Here's how the part is built. I have some questions about the finished solid (model axes, mm). Coordinates: 2 decimals unless noted, no trailing zeros. Write each loop counter-clockwise with the first axis right and the second up, starting at its lowest first coordinate (ties: lowest second). Pieces come first, ordered by that corner, then holes.
Item 1: If we section it at B-B (z = 706.5): Please give me the cut outline in (x, y), then the cut area to 3 significant figures.
Item 2: If I drill on line 1 (Y direction, x = 137, z = 936); line 2 (Y direction, x = 168, z = 928.5), over which ranges is the centre line in solid material (lowest first)?
Item 3: If we section it at A-A (x = 331.5): Please give me the cut outline in (y, z), then the cut area to 3 significant figures.
Item 4: I'm going to push flat-ended pins straight in: pin 1 Ø5 at (x, y) = (225, 2922.5) entering from -Z; pin 2 Ø1.5 at (x, y) = (300.5, 2906.5) entering from -Z; pin 3 Ø3 at (x, z) = (111, 910) entering from +Y. Where does each tip first touch, or does it pass through?
from build123d import *

# Parameters (mm, degrees)
BOSS_EXTRUDE1_DEPTH     = 3
CUT_EXTRUDE2_DEPTH      = 80
BOSS_EXTRUDE2_DEPTH     = 3
SKETCH6_R               = 4.999999998
BOSS_EXTRUDE3_DEPTH     = 3
SKETCH7_R               = 2.099999998
CUT_EXTRUDE8_DEPTH      = 103.727128927
CUT_EXTRUDE8_DEPTH_BACK = 93.470854005


with BuildPart() as part:
    # Sketch1 → Boss-Extrude1 (new body)
    with BuildSketch(Plane(origin=(349.089252495, 2874.058311474, 804.288278977), x_dir=(0.935705749, -0.202672232, 0.288753733), z_dir=(-0.118950757, -0.951829224, -0.282616075))):
        Polygon((-227.79105078, 209.509165447), (-94.070562084, 190.966487567), (-128.879732086, -60.059780262), (-262.600220782, -41.517102382), align=None)
    extrude(amount=-BOSS_EXTRUDE1_DEPTH)

    # Sketch3 → Cut-Extrude2 (cut)
    with BuildSketch(Plane(origin=(688.574610071, 446.833813903, 894.692140277), x_dir=(0.516756682, 0.537673014, -0.66623589), z_dir=(0.567103814, 0.368008283, 0.736860345))):
        Polygon((970.937778761, -219.886702224), (970.937778761, 845.245168422), (-1124.286512281, 775.631358808), (-1124.286512281, -289.500511838), align=None)
    extrude(amount=CUT_EXTRUDE2_DEPTH, mode=Mode.SUBTRACT)

    # Sketch4 → Boss-Extrude2 (add)
    with BuildSketch(Plane(origin=(357.380640452, 2859.715621096, 849.10358184), x_dir=(0.992857215, -0.11667261, -0.024940964), z_dir=(-0.118950757, -0.951829224, -0.282616075))):
        Polygon((-128.234790436, -58.388271423), (-111.076725557, -145.727367265), (1.37386057, -123.636064008), (-4.113952819, -95.701639995), align=None)
    extrude(amount=-BOSS_EXTRUDE2_DEPTH)

    # Sketch6 → Boss-Extrude3 (add)
    with BuildSketch(Plane(origin=(357.737492723, 2862.571108769, 849.951430064), x_dir=(0.992900155, -0.114030405, -0.033857781), z_dir=(0.118950757, 0.951829224, 0.282616075))):
        with Locations((-252.279251986, 111.451515819)):
            Circle(SKETCH6_R)
        with Locations((-137.453856598, 19.622629821)):
            Circle(SKETCH6_R)
        with Locations((-154.05088047, -60.894440309)):
            Circle(SKETCH6_R)
        with Locations((-96.98907211, 70.058139701)):
            Circle(SKETCH6_R)
        with Locations((-34.757829169, 88.136852409)):
            Circle(SKETCH6_R)
        with Locations((-277.861066086, -12.653428287)):
            Circle(SKETCH6_R)
    extrude(amount=-BOSS_EXTRUDE3_DEPTH)

    # Sketch7 → Cut-Extrude8 (cut, two sides)
    with BuildSketch(Plane(origin=(357.737492723, 2862.571108769, 849.951430064), x_dir=(0.992900155, -0.114030405, -0.033857781), z_dir=(0.118950757, 0.951829224, 0.282616075))) as cut_extrude8_sk:
        with Locations((-253.258660999, 111.653401888)):
            Circle(SKETCH7_R)
        with Locations((-278.8404751, -12.451542218)):
            Circle(SKETCH7_R)
        with Locations((-34.757829169, 88.136852409)):
            Circle(SKETCH7_R)
        with Locations((-96.98907211, 70.058139701)):
            Circle(SKETCH7_R)
        with Locations((-137.453856598, 19.622629821)):
            Circle(SKETCH7_R)
        with Locations((-154.05088047, -60.894440309)):
            Circle(SKETCH7_R)
    extrude(amount=CUT_EXTRUDE8_DEPTH, mode=Mode.SUBTRACT)
    extrude(cut_extrude8_sk.sketch, amount=-CUT_EXTRUDE8_DEPTH_BACK, mode=Mode.SUBTRACT)


solid = part.part
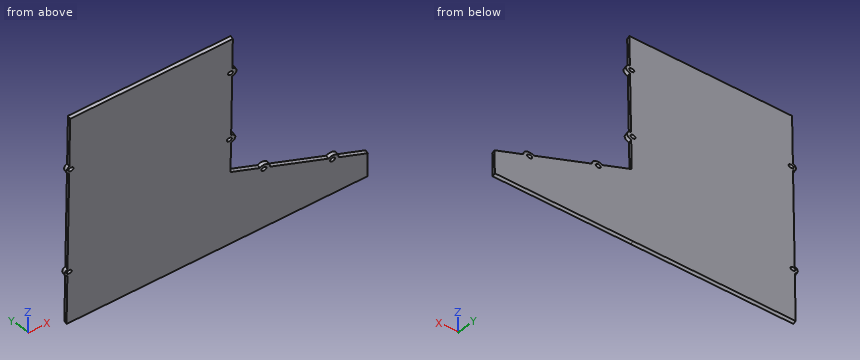
Answer list:
1. outline: (113.77, 2932.5) - (214.28, 2919.94) - (209.49, 2923.69) - (114.3, 2935.59) - close
1. area: 308 mm2
2. line 1: y = 2861.46 to 2864.61
2. line 2: y = 2859.81 to 2862.96
3. outline: (2888.05, 764.57) - (2899.55, 725.83) - (2902.47, 726.62) - (2890.92, 765.53) - close
3. area: 122 mm2
4. pin 1: stops at z = 708.61
4. pin 2: stops at z = 720.88
4. pin 3: stops at y = 2876.06
